```python
from build123d import *

# Parameters (mm, degrees)
F0_W     = 40
F0_H     = 30
F0_R     = 2
F1_DEPTH = 100
F2_R     = 1
F3_DEPTH = 30
F4_R     = 2.55
F5_DEPTH = 8
F6_R     = 1.5
F7_R     = 1.5
F8_R     = 1.5


with BuildPart() as f1:
    # F0 (on Front) → F1 (new body)
    with BuildSketch(Plane.XZ):
        Rectangle(F0_W, F0_H)
        Circle(F0_R, mode=Mode.SUBTRACT)
    extrude(amount=F1_DEPTH)

    # F2 (on face) → F3 (cut)
    with BuildSketch(Plane.XY.offset(15)):
        with Locations((0, -25)):
            Circle(F2_R)
        with Locations((0, -50)):
            Circle(F2_R)
        with Locations((0, -75)):
            Circle(F2_R)
    extrude(amount=-F3_DEPTH, mode=Mode.SUBTRACT)

    # F4 (on face) → F5 (cut)
    with BuildSketch(Plane(origin=(0, 0, -15), x_dir=(1, 0, 0), z_dir=(0, 0, -1))):
        with Locations((0, 25)):
            Circle(F4_R)
        with Locations((0, 50)):
            Circle(F4_R)
        with Locations((0, 75)):
            Circle(F4_R)
    extrude(amount=-F5_DEPTH, mode=Mode.SUBTRACT)

    # F6
    f6_edges = [f1.edges().sort_by_distance(p)[0] for p in [
        (-2.55, -25, -7),
    ]]
    fillet(f6_edges, radius=F6_R)

    # F7
    f7_edges = [f1.edges().sort_by_distance(p)[0] for p in [
        (-2.55, -50, -7),
    ]]
    fillet(f7_edges, radius=F7_R)

    # F8
    f8_edges = [f1.edges().sort_by_distance(p)[0] for p in [
        (-2.55, -75, -7),
    ]]
    fillet(f8_edges, radius=F8_R)


solid = f1.part
```
Check sheet for the modelled part. Datum: model origin and axes. Units: mm. A direction names the side the tool comes from. Round coordinates to 2 decimals unless told otherwise and drop trailing zeros. Order: outer loops, then holes, each group sorted by start corner. A loop starts at its lowest first (then second) coordinate and runs counter-clockwise, first axis right, second up. Notation, with made-up numbers: M 26,-16 L 51,-16 A25 ccw 51,13 Z; hole C 77,-30.5 d9. An arc over 180 degrees is marked long. Answer in a Markdown table with one row per item.
(1) Material ranges on line 1 along Y through (x, z) = (0, 7); line 2 along X through (y, z) = (-25, -3.4); line 3 along Z through (x, y) = (-1, -60), recorded low to high. Write a range as from..to.
Findings:
| item | result |
|---|---|
| line 1 | y = -100..-76, -74..-51, -49..-26, -24..0 |
| line 2 | x = -20..-1, 1..20 |
| line 3 | z = -15..-1.73, 1.73..15 |
(2) Draft check along Y on faces 3 (the cylindrical face through (1, -25, -4)), 4 (the flat face through (20, -49, 0)), 5 (the flat face through (0, 0, 4)). Enter one of: +Y half, -Y half, draft (parallel to the pull), parting line (faces both ways), or undercut.
Findings:
| item | result |
|---|---|
| face 3 | undercut |
| face 4 | draft |
| face 5 | +Y half |
(3) Gauge pin test, flat ends, axial feed: pin 1 (6 mm diameter, centred on x = 0, y = -25, fed in from -Z); pin 2 (2.5 mm diameter, centred on x = 0, y = -25, fed in from -Z); pin 3 (2.5 mm diameter, centred on x = 0.5, y = -25, fed in from -Z). Record the tip position at first contact, or that the pin passes through.
Findings:
| item | result |
|---|---|
| pin 1 | stops at z = -15 |
| pin 2 | stops at z = -7.01 |
| pin 3 | stops at z = -7.17 |
(4) Section check A-A on z = 0. Record the boundary of the cut face in (x, y).
Findings:
| item | result |
|---|---|
| outline | M -20,-100 L -2,-100 L -2,0 L -20,0 Z; M 2,-100 L 20,-100 L 20,0 L 2,0 Z |
(5) Set-up check for faces 1 (the cylindrical face through (-0.55, -72.51, -11.8)), 2 (the cylindrical face through (0, -26, 8)): record each of +Z, -Z, +X, -X, +Y, -Y from which the full face is reachable in a straight line by a thin tool's end or side.
Findings:
| item | result |
|---|---|
| face 1 | -Z |
| face 2 | +Z, -Z |
